Verification items for the finished model (mm, model axes). Give positions to 0.01 mm unless a question says otherwise; leave off trailing zeros. Loops run counter-clockwise (first coordinate to the right, second up) from the corner with the lowest first, then second, coordinate; pieces in that order, holes last. Notation, with made-up numbers: M 3,-25 L 54,-25 A10 cw 54,-14 Z; hole C 62.25,29 d10. An arc over 180 degrees is marked long. Answer in a Markdown table with one row per item.
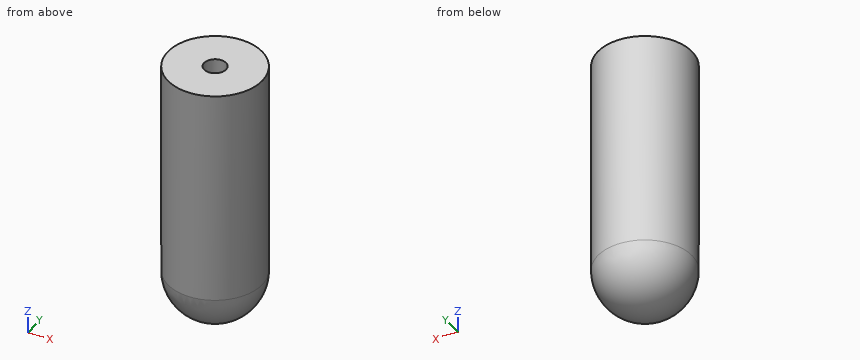
```python
from build123d import *

# Parameters (mm, degrees)
F0_R     = 14
F1_DEPTH = 64
F6_R     = 3.25
F7_DEPTH = 69.14147


# Not quite as in the source:
# - a feature of the source that left no trace in its solid (it failed there, or was rolled back) is left out


with BuildPart() as f1:
    # F0 (on Top) → F1 (new body)
    with BuildSketch(Plane.XY):
        Circle(F0_R)
    extrude(amount=F1_DEPTH)

    # F2 (on Front) → F3 (revolve)
    with BuildSketch(Plane.XZ):
        with BuildLine():
            Line((0, 0), (-14, 0))
            ThreePointArc((-14, 0), (0, -14), (14, 0))
            Line((14, 0), (0, 0))
        make_face()
    revolve(axis=Axis((0, 0, 0), (1, 0, 0)))

    # F6 (on offset) → F7 (cut)
    with BuildSketch(Plane.XY.offset(-5)):
        Circle(F6_R)
    extrude(amount=F7_DEPTH, mode=Mode.SUBTRACT)


solid = f1.part
```
Item 1: Sectioned sample at D-D (y = 9.75). Record the cut outline in (x, z), and give its area (3 significant figures).
Reported:
| item | result |
|---|---|
| outline | M -10.05,0 A10.05 ccw 10.05,0 L 10.05,64 L -10.05,64 Z |
| area | 1,440 mm^2 |
Item 2: Sectioned sample at C-C (z = 43.5). Record the cut outline in (x, y).
Reported:
| item | result |
|---|---|
| outline | C 0,0 d28; hole C 0,0 d6.5 |
Item 3: Scan lines: L1, parallel to X at y = 0, z = 34; L2, parallel to X at y = 1, z = 35.5. Record each from-to range of solid material in increasing order. Write a range as [from, to].
Reported:
| item | result |
|---|---|
| L1 | x = [-14, -3.25], [3.25, 14] |
| L2 | x = [-13.96, -3.09], [3.09, 13.96] |
Item 4: Go/stop test with flat-tipped pins: pin 1 (10.5 mm diameter, centred on x = 0, y = 0, fed in from -Z); pin 2 (10 mm diameter, centred on x = 9, z = 45, fed in from +Y); pin 3 (12 mm diameter, centred on x = 4, y = 9, fed in from -Z). Record where each tip stops, or that it passes through.
Reported:
| item | result |
|---|---|
| pin 1 | stops at z = -14 |
| pin 2 | stops at y = 13.42 |
| pin 3 | stops at z = -13.46 |
Item 5: Sectioned sample at B-B (y = -0.75). Record the cut outline in (x, z), and give its area (3 significant figures).
Reported:
| item | result |
|---|---|
| outline | M -13.98,0 A13.98 ccw 13.98,0 L 13.98,64 L 3.16,64 L 3.16,-5 L -3.16,-5 L -3.16,64 L -13.98,64 Z |
| area | 1,660 mm^2 |
Item 6: Sectioned sample at A-A (x = 0). Record the cut outline in (y, z), and give its area (3 significant figures).
Reported:
| item | result |
|---|---|
| outline | M -14,0 A14 ccw 14,0 L 14,64 L 3.25,64 L 3.25,-5 L -3.25,-5 L -3.25,64 L -14,64 Z |
| area | 1,650 mm^2 |
